For this review, take the finished solid that the model builds, in its own axes (mm). Face numbers are marked on the shaded views. A direction names the side the tool comes from. Give positions to 0.01 mm unless a question says otherwise; leave off trailing zeros. Loops run counter-clockwise (first coordinate to the right, second up) from the corner with the lowest first, then second, coordinate; pieces in that order, holes last. Notation, with made-up numbers: (24.25, -17.75) - (40.25, -17.75) arc R28 ccw to (40.25, 15.25) - close; hole circle Ø1 at (49, -4). An arc over 180 degrees is marked (long way). Put each result on its own line as item: value. Start each with the question number.
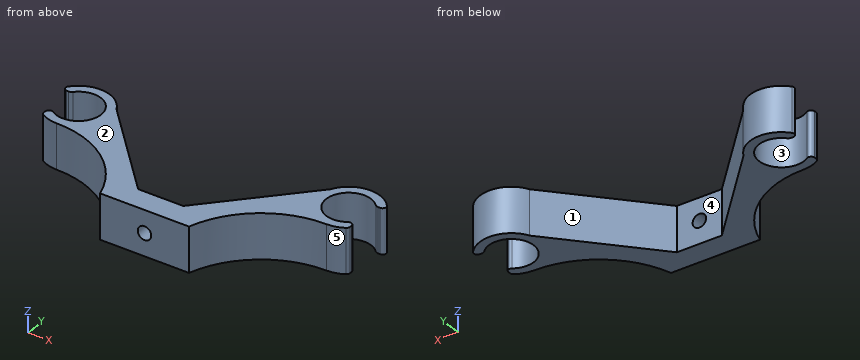
from build123d import *

# Parameters (mm, degrees)
BOSS_EXTRUDE1_DEPTH = 10
SKETCH2_R           = 1.5
CUT_EXTRUDE1_DEPTH  = 10


with BuildPart() as part:
    # Sketch1 → Boss-Extrude1 (new body)
    with BuildSketch(Plane.XY):
        with BuildLine():
            Line((9.875388203, 0), (-9.875388203, 0))
            ThreePointArc((-9.875388203, 0), (-17.450099602, 10.83745824), (-30, 15))
            ThreePointArc((-30, 15), (-31.8749625, 15.255779094), (-33.612903226, 16.004424108))
            ThreePointArc((-33.612903226, 16.004424108), (-33.896535204, 16.29613728), (-34, 16.689632781))
            Line((-34, 16.689632781), (-34, 17.162645351))
            ThreePointArc((-34, 17.162645351), (-33.578745661, 17.867309614), (-32.75862069, 17.829866682))
            ThreePointArc((-32.75862069, 17.829866682), (-25.031925557, 22.564124391), (-33.623370468, 25.445458816))
            ThreePointArc((-33.623370468, 25.445458816), (-33.953767859, 25.215558804), (-34.348044562, 25.134550579))
            Line((-34.348044562, 25.134550579), (-34.791587602, 25.134550579))
            ThreePointArc((-34.791587602, 25.134550579), (-35.51482586, 25.592605522), (-35.409856969, 26.442234524))
            ThreePointArc((-35.409856969, 26.442234524), (-29.220414383, 28.95645357), (-23.74103901, 25.134550579))
            Line((-23.74103901, 25.134550579), (-5, 5.145359938))
            Line((-5, 5.145359938), (5, 5.145359938))
            Line((5, 5.145359938), (23.74103901, 25.134550579))
            ThreePointArc((23.74103901, 25.134550579), (29.220414383, 28.95645357), (35.409856969, 26.442234524))
            ThreePointArc((35.409856969, 26.442234524), (35.51482586, 25.592605522), (34.791587602, 25.134550579))
            Line((34.791587602, 25.134550579), (34.348044562, 25.134550579))
            ThreePointArc((34.348044562, 25.134550579), (33.953767859, 25.215558804), (33.623370468, 25.445458816))
            ThreePointArc((33.623370468, 25.445458816), (25.031925557, 22.564124391), (32.75862069, 17.829866682))
            ThreePointArc((32.75862069, 17.829866682), (33.578745661, 17.867309614), (34, 17.162645351))
            Line((34, 17.162645351), (34, 16.689632781))
            ThreePointArc((34, 16.689632781), (33.896535204, 16.29613728), (33.612903226, 16.004424108))
            ThreePointArc((33.612903226, 16.004424108), (31.8749625, 15.255779094), (30, 15))
            ThreePointArc((30, 15), (17.450099602, 10.83745824), (9.875388203, 0))
        make_face()
    extrude(amount=BOSS_EXTRUDE1_DEPTH)

    # Sketch2 → Cut-Extrude1 (cut)
    with BuildSketch(Plane(origin=(0, 5.145359938, 0), x_dir=(1, 0, 0), z_dir=(0, 1, 0))):
        with Locations((0, -5)):
            Circle(SKETCH2_R)
    extrude(amount=-CUT_EXTRUDE1_DEPTH, mode=Mode.SUBTRACT)


solid = part.part
1) Take a section at A-A on x = 0. State the section outline as (y, z) points, and give its area (3 significant figures).
2) Machinability: for the marked faces 1 and 2, which of the approach directions +Z, -Z, +X, -X, +Y, -Y give a long, thin tool a straight path to every point of the face, cutting with its end or side? Answer none if there is none.
3) Wall thickness on probe 1 along Y at (x, z) = (30, 7); probe 2 along Z at (x, y) = (0, 2.8); probe 3 along X at (y, z) = (25, 4.5): over which ranges is each line inside the solid? List them lowest first.
4) Take a section at C-C on z = 5. State the section outline as (x, y) points, and give its area (3 significant figures).
5) Insertion check: P1, Ø0.5, axis at y = 17, z = 6.5, coming from the +X side; P2, Ø5, axis at y = 8.5, z = 8, coming from the -X side; P3, Ø1.5, axis at x = -0.5, z = 1.5, coming from the +Y side. Each pin has a flat end and moves straight along its axis. Give the tip position at first contact, or say it passes through.
6) Take a section at B-B on y = 21.5. State the section outline as (x, z) points.
7) Take a section at D-D on x = -8.5. State the section outline as (y, z) points.
8) Mouldability with a two-part tool opening along Y and no side actions: class the marked faces 3, 4 and 5 as released by +Y, released by -Y, zero draft, split by the parting line, or undercut.
Answers follow:
1. outline: (0, 0) - (5.15, 0) - (5.15, 3.5) - (0, 3.5) - close; (0, 6.5) - (5.15, 6.5) - (5.15, 10) - (0, 10) - close
1. area: 36.0 mm2
2. face 1: +Z, -Z, +Y
2. face 2: +Z, +X, -X, +Y, -Y
3. probe 1: 15 to 17, 27 to 29
3. probe 2: 0 to 3.5, 6.5 to 10
3. probe 3: -26 to -23.61, 23.61 to 26
4. outline: (-35.41, 26.44) arc R0.8 ccw to (-34.79, 25.13) - (-34.35, 25.13) arc R1 ccw to (-33.62, 25.45) arc R5 cw (long way) to (-32.76, 17.83) arc R0.8 ccw to (-34, 17.16) - (-34, 16.69) arc R0.8 ccw to (-33.61, 16) arc R7 ccw to (-30, 15) arc R21 cw to (-9.88, 0) - (-1.5, 0) - (-1.5, 5.15) - (-5, 5.15) - (-23.74, 25.13) arc R7 ccw to start; (1.5, 0) - (9.88, 0) arc R21 cw to (30, 15) arc R7 ccw to (33.61, 16) arc R0.8 ccw to (34, 16.69) - (34, 17.16) arc R0.8 ccw to (32.76, 17.83) arc R5 cw (long way) to (33.62, 25.45) arc R1 ccw to (34.35, 25.13) - (34.79, 25.13) arc R0.8 ccw to (35.41, 26.44) arc R7 ccw to (23.74, 25.13) - (5, 5.15) - (1.5, 5.15) - close
4. area: 470 mm2
5. P1: x = 34
5. P2: x = -17.67
5. P3: y = 5.15
6. outline: (-25.03, 0) - (-20.33, 0) - (-20.33, 10) - (-25.03, 10) - close; (20.33, 0) - (25.03, 0) - (25.03, 10) - (20.33, 10) - close
7. outline: (0, 0) - (8.88, 0) - (8.88, 10) - (0, 10) - close
8. face 3: undercut
8. face 4: released by +Y
8. face 5: released by -Y
